Model file for the job. Use its own axes, mm. Give positions to 0.01 mm unless a question says otherwise; leave off trailing zeros. Order: outer loops, then holes, each group sorted by start corner. A loop starts at its lowest first (then second) coordinate and runs counter-clockwise, first axis right, second up. Notation, with made-up numbers: (85.25, 6.5) - (93.25, 6.5) arc R27 cw to (93.25, 42.5) - close; hole circle Ø9 at (62, 59). An arc over 180 degrees is marked (long way). Use CSV: the item, a comma, the result in double quotes. Start each with the question number.
(1) Probe L1, parallel to Y at x = 1, z = -78.5 (3 decimals); L2, parallel to Y at x = 8.75, z = 87 (3 decimals). List the from-to ranges inside material, lowest first.
(2) Band-saw the part on B-B, the plane x = -2.5. Give the cut face in (y, z) (3 decimals).
(3) Drop flat-ended pins along their axis: pin 1 Ø8 at (x, z) = (-3, 39.5) entering from +Y (3 decimals); pin 2 Ø1 at (x, z) = (-7, -7) entering from +Y (3 decimals); pin 3 Ø4 at (x, z) = (-2, -73.5) entering from +Y (3 decimals). Give the stop position or say it passes through.
from build123d import *

# Parameters (mm, degrees)
F0_W     = 9.525
F0_H     = 95.25
F1_DEPTH = 457.2
F2_SIZE  = 19.04999


# Not quite as in the source:
# - a fillet or chamfer is up to 0.001 mm smaller than in the source, because OpenCascade refuses the exact size


with BuildPart() as f1:
    # F0 (on Front) → F1 (new body, symmetric)
    with BuildSketch(Plane.XZ):
        Polygon((9.525, 95.25), (-9.525, 95.25), (-9.525, 0), (0, 0), (9.525, 0), align=None)
        with Locations((-4.7625, -47.625)):
            Rectangle(F0_W, F0_H)
        with Locations((4.7625, -47.625)):
            Rectangle(F0_W, F0_H)
    extrude(amount=F1_DEPTH, both=True)

    # F2 (size 19.05 in the source; OpenCascade refuses exactly that, so slightly less here)
    f2_edges = [f1.edges().sort_by_distance(p)[0] for p in [
        (9.525, -457.2, 0),
        (9.525, 457.2, 0),
    ]]
    chamfer(f2_edges, length=F2_SIZE)


solid = f1.part
Answer block:
1,L1,"y = -446.675 to 446.675"
1,L2,"y = -438.925 to 438.925"
2,outline,"(-450.175, -95.25) - (450.175, -95.25) - (450.175, 95.25) - (-450.175, 95.25) - close"
3,pin 1,"stops at y = 454.675"
3,pin 2,"stops at y = 455.175"
3,pin 3,"stops at y = 451.675"
